Work out the finished part from the listing and answer in its coordinate system (mm). Give positions to 0.01 mm unless a question says otherwise; leave off trailing zeros. Order: outer loops, then holes, each group sorted by start corner. A loop starts at its lowest first (then second) coordinate and runs counter-clockwise, first axis right, second up. Notation, with made-up numbers: (-5, 3.25) - (44, 3.25) arc R26 ccw to (44, 30.25) - close; hole circle Ø3 at (82.5, 12.25). An arc over 180 degrees is marked (long way). Write each question's results on one line, items separated by ' | '.
Autodesk Inventor part; units mm, degrees
ref_plane "YZ Plane" through (0, 0, 0) normal (1, 0, 0) x (0, 1, 0)
ref_plane "XZ Plane" through (0, 0, 0) normal (0, 1, 0) x (-1, 0, 0)
ref_plane "XY Plane" through (0, 0, 0) normal (0, 0, 1) x (1, 0, 0)
sketch "Esboço1" plane through (0, 0, 0) normal (0, 0, 1) x (1, 0, 0)
  line L0 (-3, 20) -> (0, 20)
  line L1 (-3, 20) -> (-3, 18)
  line L2 (-3, 18) -> (-2, 18)
  line L3 (-2, 18) -> (-2, 1)
  line L4 (-2, 1) -> (-7, 1)
  line L5 (-7, 1) -> (-7, 0)
  line L6 (-7, 0) -> (0, 0)
  line L7 (0, 20) -> (0, 0)
  line L8 (-8.4, 0) -> (1.4, 0)
  line L9 (0, -4) -> (0, 24)
  dimension "d0" = 20
  dimension "d1" = 3
  dimension "d2" = 2
  dimension "d3" = 1
  dimension "d4" = 5
  dimension "d5" = 1
revolve "Revolução1" add sketch "Esboço1" angle 360 about axis through (0, -10, 0) along (0, 1, 0)
sketch "Esboço2" plane through (0, 0, 0) normal (0, 0, 1) x (1, 0, 0)
  line L0 (-2.5, 0) -> (2.5, 0)
  line L1 (2.5, 0) -> (2.5, -100)
  line L2 (2.5, -100) -> (2.5, -64.1353)
  arc A0 (-2.5, -91.3397) -> (2.5, -100) centre (7.5, -91.3397) ccw
  line L3 (-2.5, 0) -> (-2.5, -91.3397)
  line L4 (7, 0) -> (-7, 0)
  point P0 (0, 0)
  point P1 (0, 0)
  dimension "d7" = 100
  dimension "d8" = 5
  dimension "d10" = 10
extrude "Extrusão1" add sketch "Esboço2" along normal mid plane 1
fillet "Arredondamento1" radius 2 2 edges at (-1.1603, -96.3397, 0.5) (-2.5, -45.6699, 0.5)
properties part number "katana"
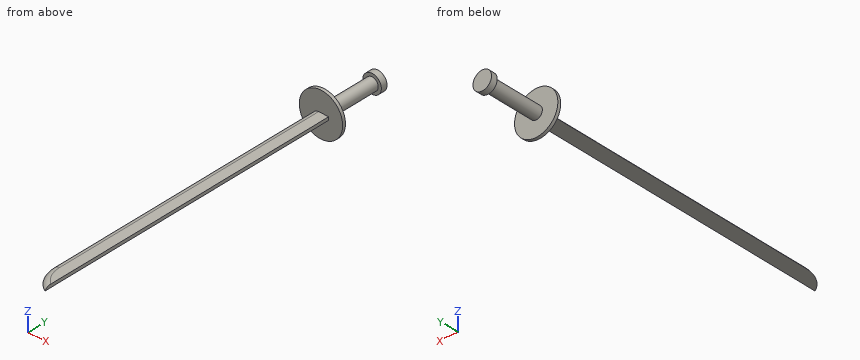
1. A cutting plane is placed at A-A, the plane y = 12. Write down the section's boundary in (x, z).
Answer list:
outline: circle Ø4 at (0, 0)
2. A cutting plane is placed at B-B, the plane x = 5.25. Write down the section's boundary in (y, z).
Answer list:
outline: (0, -4.63) - (1, -4.63) - (1, 4.63) - (0, 4.63) - close
3. A cutting plane is placed at C-C, the plane z = 5.75. Write down the section's boundary in (x, y).
Answer list:
outline: (-3.99, 0) - (3.99, 0) - (3.99, 1) - (-3.99, 1) - close
4. Straight lines are drawn through the part: line 1 (Y direction, x = -2, z = -1.25); line 2 (Z direction, x = -0.75, y = -86); line 3 (Y direction, x = -1, z = -6). For each, find the intervals that lie inside material, in ascending order. Write a range as [from, to].
Answer list:
line 1: [0, 1], [18, 20] | line 2: [-0.5, 0.5] | line 3: [0, 1]
5. Given P1, Ø0.5, axis at y = -26.5, z = 0, coming from the +X side; P2, Ø1, axis at x = 2.5, z = -2, coming from the +Y side; P3, Ø1, axis at x = 3, z = 2.5, coming from the +Y side; P4, Ø1.5, axis at x = -3.5, z = -0.5, coming from the -Y side, each flat-ended and moving along its own axis, determine where each tip first touches the part or whether it passes through.
Answer list:
P1: x = 2.5 | P2: y = 20 | P3: y = 1 | P4: y = 0
